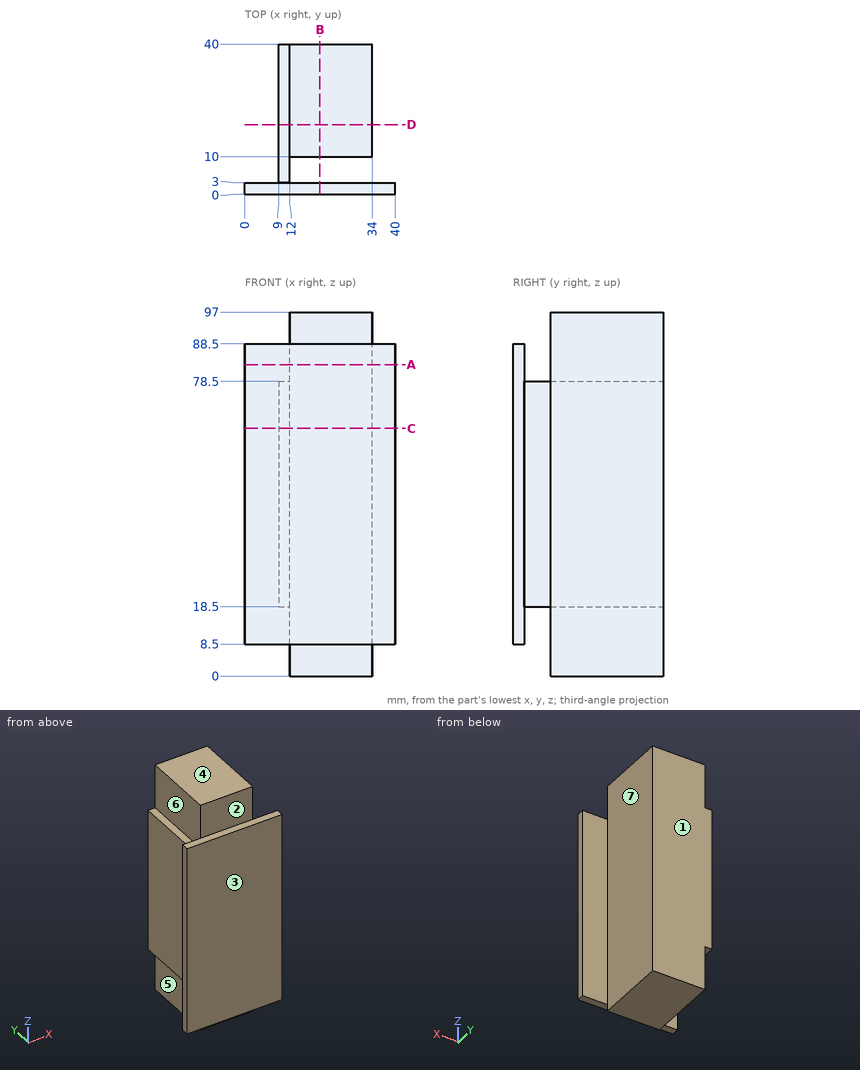
For this review, use the dimensioned drawing (mm, ordinates from the lowest corner) and the shaded views. A direction names the side the tool comes from. Round coordinates to 2 decimals unless told otherwise and drop trailing zeros. Order: outer loops, then holes, each group sorted by start corner. A loop starts at its lowest first (then second) coordinate and runs counter-clockwise, first axis right, second up. Notation, with made-up numbers: (56.5, 12) -> (100.5, 12) arc R27 ccw to (100.5, 51) -> close; hole circle Ø9 at (-27, 24). An arc over 180 degrees is marked (long way). One line per item, written item: value. Start each with the question number.
Q1. Machinability: for the marked faces 5, 6 and 7, which of the approach directions +Z, -Z, +X, -X, +Y, -Y give a long, thin tool a straight path to every point of the face, cutting with its end or side? Answer none if there is none.
Q2. Take a section at C-C (z = 66). Write out the cut boundary in (x, y), and give its area (3 significant figures).
Q3. Clearance check with flat-ended pins moving along their axes: pin 1 Ø5.5 at (y, z) = (18, 6) entering from -X; pin 2 Ø10 at (y, z) = (9, 43) entering from +X; pin 3 Ø8 at (y, z) = (18, 60.5) entering from -X. State where each tip first meets the part, or that it passes through.
Q4. Take a section at A-A (z = 83). Write out the cut boundary in (x, y).
Q5. Wall thickness on line 1 (Y direction, x = 19.5, z = 65.5); line 2 (X direction, y = 11, z = 29); line 3 (Y direction, x = 11, z = 80): over which ranges is each line inside the solid? List them lowest first.
Q6. Take a section at D-D (y = 18.5). Write out the cut boundary in (x, z).
Q7. Take a section at B-B (x = 20). Write out the cut boundary in (y, z), and give its area (3 significant figures).
Q8. Mouldability with a two-part tool opening along Y and no side actions: class the marked faces 1, 2, 3 and 4 as released by +Y, released by -Y, zero draft, split by the parting line, or undercut.
Reported:
1. face 5: -Z, -X, +Y
1. face 6: +Z, -X, +Y
1. face 7: +Z, -Z, +X, +Y
2. outline: (0, 0) -> (40, 0) -> (40, 3) -> (12, 3) -> (12, 10) -> (34, 10) -> (34, 40) -> (9, 40) -> (9, 3) -> (0, 3) -> close
2. area: 891 mm2
3. pin 1: stops at x = 12
3. pin 2: stops at x = 34
3. pin 3: stops at x = 9
4. outline: (0, 0) -> (40, 0) -> (40, 3) -> (0, 3) -> close; (12, 10) -> (34, 10) -> (34, 40) -> (12, 40) -> close
5. line 1: y = 0 to 3, 10 to 40
5. line 2: x = 9 to 34
5. line 3: y = 0 to 3
6. outline: (9, 18.5) -> (12, 18.5) -> (12, 0) -> (34, 0) -> (34, 97) -> (12, 97) -> (12, 78.5) -> (9, 78.5) -> close
7. outline: (0, 8.5) -> (3, 8.5) -> (3, 88.5) -> (0, 88.5) -> close; (10, 0) -> (40, 0) -> (40, 97) -> (10, 97) -> close
7. area: 3,150 mm2
8. face 1: released by +Y
8. face 2: undercut
8. face 3: released by -Y
8. face 4: zero draft
